Can you work these out from the model? Positions are in its coordinate system, mm. Face numbers are marked on the shaded views. Round coordinates to 2 decimals unless told otherwise and drop trailing zeros. Order: outer loops, then holes, each group sorted by start corner. A loop starts at its lowest first (then second) coordinate and runs counter-clockwise, first axis right, second up. Notation, with made-up numbers: M 43.25,-17.5 L 87.25,-17.5 A19 cw 87.25,-7.5 Z; hole C 87.25,48.5 d4. An arc over 180 degrees is marked long. Answer as a JSON object with one key per item and string values. Group by question number.
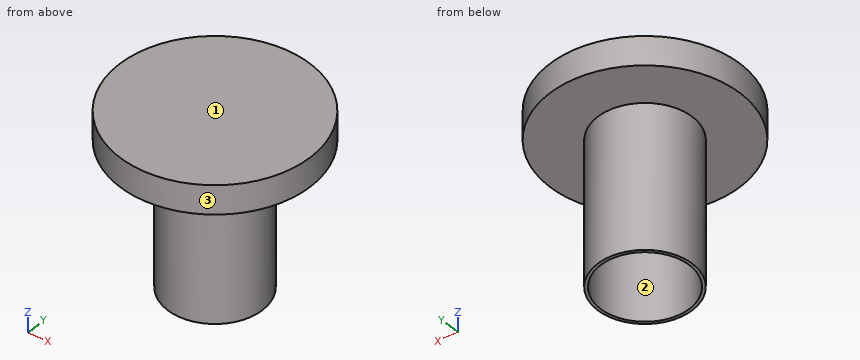
```python
from build123d import *

# Parameters (mm, degrees)
F2_R     = 16.5
F3_DEPTH = 5
F4_R     = 8.2
F4_R_2   = 7.7
F5_DEPTH = 25


# Not quite as in the source:
# - the program builds the solid bodies; features that only make, move or delete a surface that nothing else refers to are left out


with BuildPart() as f3:
    # F2 (on Top) → F3 (new body)
    with BuildSketch(Plane.XY):
        with Locations((-45.8642121462, 17.7900076957)):
            Circle(F2_R)
    extrude(amount=F3_DEPTH)

    # F4 (on Top) → F5 (join)
    with BuildSketch(Plane.XY):
        with Locations((-45.8642121462, 17.7900076957)):
            Circle(F4_R)
        with Locations((-45.8642121462, 17.7900076957)):
            Circle(F4_R_2, mode=Mode.SUBTRACT)
    extrude(amount=-F5_DEPTH)


solid = f3.part
```
1) I need wall thicknesses on line 1 along Z through (x, y) = (-57, 15); line 2 along X through (y, z) = (14, -18.5); line 3 along X through (y, z) = (22.5, -10). Which ranges of each line are inside material? Lowest first, please.
2) If we section it at C-C on z = -2.5: Write out the boundary of the cut face in (x, y), plus the area to 3 significant figures.
3) If we section it at B-B on y = 23: Write out the boundary of the cut face in (x, z).
4) We'd pull the mould along Y, two halves only. Please class the marked faces 1, 2 and 3: +Y half, -Y half, draft (parallel to the pull), parting line (faces both ways), or undercut.
5) If we section it at A-A on x = -47: Write out the boundary of the cut face in (y, z), plus the area to 3 significant figures.
6) If we section it at D-D on y = 28.5: Write out the boundary of the cut face in (x, z).
7) For pin 1 (2 mm diameter, centred on y = 24, z = 0, fed in from +X); pin 2 (1.5 mm diameter, centred on y = 22.5, z = -2.5, fed in from -X); pin 3 (1 mm diameter, centred on x = -45, y = 17.5, fed in from -Z), each with a flat end and sliding along its axis, tell me the tip position at first contact or that it passes through.
Findings:
{
 "1": {"line 1": "z = 0 to 5", "line 2": "x = -53.14 to -52.57, -39.16 to -38.59", "line 3": "x = -52.58 to -51.96, -39.77 to -39.15"},
 "2": {"outline": "C -45.86,17.79 d16.4; hole C -45.86,17.79 d15.4", "area": "25.0 mm^2"},
 "3": {"outline": "M -61.52,0 L -52.2,0 L -52.2,-25 L -51.53,-25 L -51.53,0 L -40.19,0 L -40.19,-25 L -39.53,-25 L -39.53,0 L -30.21,0 L -30.21,5 L -61.52,5 Z"},
 "4": {"face 1": "draft", "face 2": "undercut", "face 3": "parting line"},
 "5": {"outline": "M 1.33,0 L 9.67,0 L 9.67,-25 L 10.17,-25 L 10.17,0 L 25.41,0 L 25.41,-25 L 25.91,-25 L 25.91,0 L 34.25,0 L 34.25,5 L 1.33,5 Z", "area": "190 mm^2"},
 "6": {"outline": "M -58.42,0 L -33.31,0 L -33.31,5 L -58.42,5 Z"},
 "7": {"pin 1": "stops at x = -30.21", "pin 2": "stops at x = -53.04", "pin 3": "stops at z = 0"}
}
